Source: CAD feature listing. Evaluate the final solid. Frame: model axes, mm. Face numbers are marked on the shaded views. A direction names the side the tool comes from. Give positions to 0.01 mm unless a question says otherwise; leave off trailing zeros. Loops run counter-clockwise (first coordinate to the right, second up) from the corner with the lowest first, then second, coordinate; pieces in that order, holes last. Notation, with made-up numbers: (-16, 41.25) - (8, 41.25) arc R12 ccw to (8, 64.25) - close; hole circle Ø8 at (19, 22.5). An arc over 180 degrees is marked (long way). Write each question's results on one line, items separated by ' | '. Start each with the question number.
(1) Cut plane B-B on x = -29. Return the cut outline in (y, z).
(2) Material intervals for line 1 along X through (y, z) = (3.25, 0.5); line 2 along Z through (x, y) = (-26, -0.5); line 3 along Z through (x, y) = (-34.5, 0.5), sorted ascending. Write a range as [from, to].
(3) Cut plane A-A on x = -3. Return the cut outline in (y, z), then the cut area to 3 significant figures.
(4) Pull-direction query (X, two-part tool) for the marked faces 1, 2 and 3; classes: pulls with the +X half, pulls with the -X half, needs draft (parallel to the pull), parting line crosses it, or undercut.
(5) Reachability of the marked faces 4, 5 and 6 from +Z, -Z, +X, -X, +Y, -Y: full face, straight path, thin tool, end or side. Return the list, or none.
(6) Contact query for flat-ended pins moving along their axis: pin 1 (2 mm diameter, centred on x = -6, z = -1, fed in from -Y); pin 2 (5 mm diameter, centred on x = -33, z = -0.5, fed in from -Y); pin 3 (1.5 mm diameter, centred on x = -17.5, y = 3, fed in from +Z). Output: stop coordinate, or through.
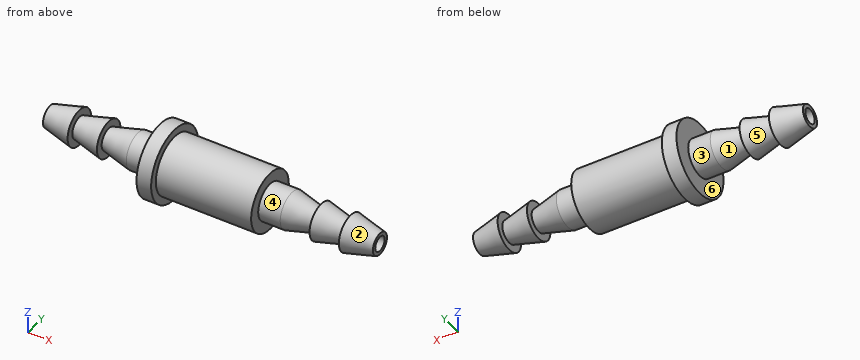
from build123d import *

# Parameters (mm, degrees)
SKETCH_2_R          = 1
CUT_EXTRUDE_1_DEPTH = 46


with BuildPart() as part:
    # Эскиз1 → Повернуть1 (revolve)
    with BuildSketch(Plane.XY):
        Polygon((-30, 2.5), (-33, 2.5), (-37, 1.5), (-37, 2.5), (-41, 1.5), (-41, 2.5), (-45, 1.5), (-45, 0), (0, 0), (0, 1.5), (-4, 2.5), (-4, 1.5), (-8, 2.5), (-8, 1.5), (-12, 2.5), (-15, 2.5), (-15, 4), (-28, 4), (-28, 5), (-30, 5), align=None)
    revolve(axis=Axis((-45, 0, 0), (1, 0, 0)))

    # Эскиз2 → Вырез-Вытянуть1 (cut, through all)
    with BuildSketch(Plane.ZY.offset(45)):
        Circle(SKETCH_2_R)
    extrude(amount=-CUT_EXTRUDE_1_DEPTH, mode=Mode.SUBTRACT)


solid = part.part
Ans:
1) outline: circle Ø10 at (0, 0); hole circle Ø2 at (0, 0)
2) line 1: [-30, -15] | line 2: [-3.97, -0.87], [0.87, 3.97] | line 3: [-2.07, -0.87], [0.87, 2.07]
3) outline: circle Ø4.5 at (0, 0); hole circle Ø2 at (0, 0) | area: 12.8 mm^2
4) face 1: undercut | face 2: pulls with the +X half | face 3: needs draft
5) face 4: +X | face 5: none | face 6: -X
6) pin 1: y = -2.16 | pin 2: y = -2.5 | pin 3: z = 3.31
